Check sheet for the modelled part. Datum: model origin and axes. Units: mm. Face numbers are marked on the shaded views. A direction names the side the tool comes from. Round coordinates to 2 decimals unless told otherwise and drop trailing zeros. Write each loop counter-clockwise with the first axis right and the second up, starting at its lowest first coordinate (ties: lowest second). Pieces come first, ordered by that corner, then holes. Notation, with made-up numbers: M -8,46 L 10,46 A20 cw 10,65 Z; hole C 28,-39.75 d10. An arc over 180 degrees is marked long. Answer in a Markdown table with one row per item.
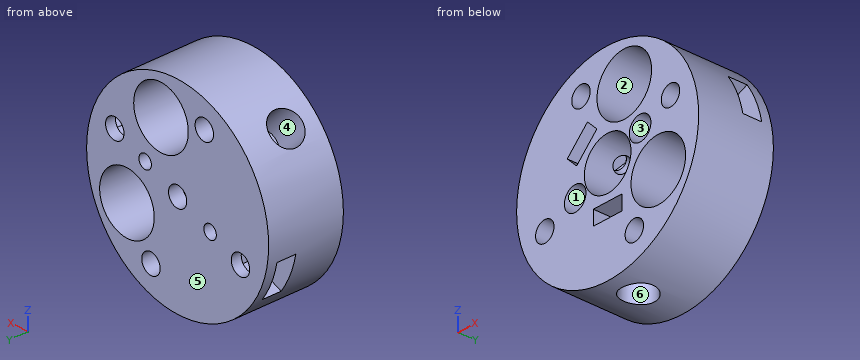
```python
from build123d import *

# Parameters (mm, degrees)
SKETCH1_R               = 20
BOSS_EXTRUDE1_DEPTH     = 7.5
SKETCH4_R               = 5.125
CUT_EXTRUDE2_DEPTH      = 12.15
SKETCH5_R               = 2
CUT_EXTRUDE3_DEPTH      = 1
CUT_EXTRUDE3_DEPTH_BACK = 16
SKETCH2_R               = 2.025
CUT_EXTRUDE1_DEPTH      = 16
CIRPATTERN1_COUNT       = 4
SKETCH6_R               = 1.525
CUT_EXTRUDE4_DEPTH      = 21
CUT_EXTRUDE5_START      = -20
SKETCH7_R               = 3.25
CUT_EXTRUDE5_DEPTH      = 8
CUT_EXTRUDE11_START     = -6.5
CUT_EXTRUDE11_DEPTH     = 2.9
CIRPATTERN2_COUNT       = 2
CIRPATTERN2_ANGLE       = 135
CUT_EXTRUDE7_START      = 5.5
CUT_EXTRUDE7_DEPTH      = 3.8
CIRPATTERN3_COUNT       = 2
CUT_EXTRUDE12_START     = -16.0000001
SKETCH10_R              = 6
CUT_EXTRUDE12_DEPTH     = 17.0000002
CIRPATTERN4_COUNT       = 2
CIRPATTERN4_ANGLE       = 100
CUT_EXTRUDE13_START     = -16.0000001
SKETCH11_R              = 1.375
CUT_EXTRUDE13_DEPTH     = 17.0000002
SKETCH13_R              = 2.375
CUT_EXTRUDE24_DEPTH     = 12
CIRPATTERN5_COUNT       = 2


with BuildPart() as part:
    # Sketch1 → Boss-Extrude1 (new body, symmetric)
    with BuildSketch(Plane(origin=(0, 0, 0), x_dir=(1, 0, 0), z_dir=(0, 1, 0))):
        Circle(SKETCH1_R)
    extrude(amount=BOSS_EXTRUDE1_DEPTH, both=True)

    # Sketch4 → Cut-Extrude2 (cut)
    with BuildSketch(Plane.XZ.offset(7.5)):
        Circle(SKETCH4_R)
    extrude(amount=-CUT_EXTRUDE2_DEPTH, mode=Mode.SUBTRACT)

    # Sketch5 → Cut-Extrude3 (cut, two sides)
    with BuildSketch(Plane(origin=(0, 7.5, 0), x_dir=(1, 0, 0), z_dir=(0, 1, 0))) as cut_extrude3_sk:
        Circle(SKETCH5_R)
    extrude(amount=CUT_EXTRUDE3_DEPTH, mode=Mode.SUBTRACT)
    extrude(cut_extrude3_sk.sketch, amount=-CUT_EXTRUDE3_DEPTH_BACK, mode=Mode.SUBTRACT)

    # Sketch2 → Cut-Extrude1 (cut, through all)
    with BuildSketch(Plane(origin=(0, 7.5, 0), x_dir=(1, 0, 0), z_dir=(0, 1, 0))):
        with Locations((-13.807572802, 5.860966927)):
            Circle(SKETCH2_R)
    cut_extrude1 = extrude(amount=-CUT_EXTRUDE1_DEPTH, mode=Mode.SUBTRACT)

    # CirPattern1: Cut-Extrude1 ×4 about axis
    cirpattern1_axis = Axis((0, 0, 0), (0, 1, 0))
    for i in range(1, CIRPATTERN1_COUNT):
        add(cut_extrude1.rotate(cirpattern1_axis, i * 360 / CIRPATTERN1_COUNT), mode=Mode.SUBTRACT)

    # Sketch6 → Cut-Extrude4 (cut, through all)
    with BuildSketch(Plane.XY):
        with Locations((0, -1.35)):
            Circle(SKETCH6_R)
    cut_extrude4 = extrude(amount=-CUT_EXTRUDE4_DEPTH, mode=Mode.SUBTRACT)

    # Sketch7 → Cut-Extrude5 (cut)
    with BuildSketch(Plane.XY.offset(CUT_EXTRUDE5_START)):
        with Locations((0, -1.35)):
            Circle(SKETCH7_R)
    cut_extrude5 = extrude(amount=CUT_EXTRUDE5_DEPTH, mode=Mode.SUBTRACT)

    # Sketch9 → Cut-Extrude11 (cut)
    with BuildSketch(Plane.XY.offset(CUT_EXTRUDE11_START)):
        Polygon((3.15, -3.168653348), (3.15, 0.468653348), (0, 2.287306696), (-3.15, 0.468653348), (-3.15, -3.168653348), (-3.15, -7.685074736), (3.15, -7.685074736), align=None)
    cut_extrude11 = extrude(amount=-CUT_EXTRUDE11_DEPTH, mode=Mode.SUBTRACT)

    # CirPattern2: Cut-Extrude4, Cut-Extrude5, Cut-Extrude11 ×2 about axis
    cirpattern2_axis = Axis((0, 0, 0), (0, 1, 0))
    for i in range(1, CIRPATTERN2_COUNT):
        add(cut_extrude4.rotate(cirpattern2_axis, i * CIRPATTERN2_ANGLE / (CIRPATTERN2_COUNT - 1)), mode=Mode.SUBTRACT)
        add(cut_extrude5.rotate(cirpattern2_axis, i * CIRPATTERN2_ANGLE / (CIRPATTERN2_COUNT - 1)), mode=Mode.SUBTRACT)
        add(cut_extrude11.rotate(cirpattern2_axis, i * CIRPATTERN2_ANGLE / (CIRPATTERN2_COUNT - 1)), mode=Mode.SUBTRACT)

    # Sketch8 → Cut-Extrude7 (cut)
    with BuildSketch(Plane(origin=(0, 0, 0), x_dir=(1, 0, 0), z_dir=(0, 1, 0)).offset(CUT_EXTRUDE7_START)):
        Polygon((-9.396506885, 3.988580533), (-9.98050566, 8.744868872), (-14.391571577, 10.617255266), (-19.569899143, 12.815324908), (-22.81296751, 5.175134625), (-17.634639943, 2.977064983), (-13.223574027, 1.104678588), align=None)
    cut_extrude7 = extrude(amount=-CUT_EXTRUDE7_DEPTH, mode=Mode.SUBTRACT)

    # CirPattern3: Cut-Extrude7 ×2 about axis
    cirpattern3_axis = Axis((0, 0, 0), (0, 1, 0))
    for i in range(1, CIRPATTERN3_COUNT):
        add(cut_extrude7.rotate(cirpattern3_axis, i * 360 / CIRPATTERN3_COUNT), mode=Mode.SUBTRACT)

    # Sketch10 → Cut-Extrude12 (cut)
    with BuildSketch(Plane(origin=(0, 7.5, 0), x_dir=(1, 0, 0), z_dir=(0, 1, 0)).offset(CUT_EXTRUDE12_START)):
        with Locations((3.654646309, -11.95380945)):
            Circle(SKETCH10_R)
    cut_extrude12 = extrude(amount=CUT_EXTRUDE12_DEPTH, mode=Mode.SUBTRACT)

    # CirPattern4: Cut-Extrude12 ×2 about axis
    cirpattern4_axis = Axis((0, 7.5, 0), (0, 1, 0))
    for i in range(1, CIRPATTERN4_COUNT):
        add(cut_extrude12.rotate(cirpattern4_axis, i * CIRPATTERN4_ANGLE / (CIRPATTERN4_COUNT - 1)), mode=Mode.SUBTRACT)

    # Sketch11 → Cut-Extrude13 (cut)
    with BuildSketch(Plane(origin=(0, 7.5, 0), x_dir=(1, 0, 0), z_dir=(0, 1, 0)).offset(CUT_EXTRUDE13_START)):
        with Locations((7.133912614, -3.028166246)):
            Circle(SKETCH11_R)
    cut_extrude13 = extrude(amount=CUT_EXTRUDE13_DEPTH, mode=Mode.SUBTRACT)

    # Sketch13 → Cut-Extrude24 (cut)
    with BuildSketch(Plane(origin=(0, -7.5, 0), x_dir=(-1, 0, 0), z_dir=(0, -1, 0))):
        with Locations((-7.133912614, -3.028166246)):
            Circle(SKETCH13_R)
    cut_extrude24 = extrude(amount=-CUT_EXTRUDE24_DEPTH, mode=Mode.SUBTRACT)

    # CirPattern5: Cut-Extrude13, Cut-Extrude24 ×2 about axis
    cirpattern5_axis = Axis((0, 0, 0), (0, 1, 0))
    for i in range(1, CIRPATTERN5_COUNT):
        add(cut_extrude13.rotate(cirpattern5_axis, i * 360 / CIRPATTERN5_COUNT), mode=Mode.SUBTRACT)
        add(cut_extrude24.rotate(cirpattern5_axis, i * 360 / CIRPATTERN5_COUNT), mode=Mode.SUBTRACT)


solid = part.part
```
1. Section check B-B, the plane y = -5.25. Count the separate pieces of the cut face and the enclosed holes in it, and give its area (3 significant figures).
Found:
| item | result |
|---|---|
| separate pieces | 1 |
| enclosed holes | 11 |
| area | 824 mm2 |
2. Section check C-C, the plane x = 12.5. Record the cut outline in (y, z).
Found:
| item | result |
|---|---|
| outline | M -7.5,-15.61 L 7.5,-15.61 L 7.5,-11.52 L -7.5,-11.52 Z; M -7.5,0.17 L 7.5,0.17 L 7.5,4.31 L 5.5,4.31 L 5.5,1.65 L 1.7,1.65 L 1.7,4.31 L -7.5,4.31 Z; M -7.5,7.41 L 1.7,7.41 L 1.7,9.81 L 5.5,9.81 L 5.5,7.41 L 7.5,7.41 L 7.5,15.61 L -7.5,15.61 Z |
3. Go/stop test with flat-tipped pins: pin 1 (1.5 mm diameter, centred on x = 8, y = 5.5, fed in from +Z); pin 2 (6 mm diameter, centred on y = 1, z = 6.5, fed in from +X); pin 3 (5 mm diameter, centred on x = -3.5, y = -2, fed in from +Z) (3 decimals). Record where each tip stops, or that it passes through.
Found:
| item | result |
|---|---|
| pin 1 | stops at z = 18.64 |
| pin 2 | stops at x = 19.69 |
| pin 3 | stops at z = 19.975 |
4. Scan lines: L1, parallel to Y at x = 16, z = 7; L2, parallel to Z at x = 2, y = 0.25; L3, parallel to Z at x = 16, y = 4.5. Record each from-to range of solid material in increasing order.
Found:
| item | result |
|---|---|
| L1 | y = -7.5 to 1.7, 5.5 to 7.5 |
| L2 | z = -12 to -9.4, -6.5 to -4.72, 4.72 to 6.19, 17.72 to 19.9 |
| L3 | z = -12 to -9.19, -2.16 to 2.28, 11.3 to 12 |
5. Access from +Z, -Z, +X, -X, +Y, -Y to the whole of each face (thin tool, end or side, straight path). Record for the marked faces 1 and 2.
Found:
| item | result |
|---|---|
| face 1 | -Y |
| face 2 | +Y, -Y |
6. Section check A-A, the plane z = -15. Record the cut outline in (x, y).
Found:
| item | result |
|---|---|
| outline | M -13.23,-7.5 L 4.22,-7.5 L 4.22,7.5 L -13.23,7.5 Z; M 7.5,-7.5 L 13.23,-7.5 L 13.23,7.5 L 7.5,7.5 Z; hole C 0,-1.35 d6.5 |
7. Draft check along Y on the marked faces 3, 4, 5 and 6. Enter one of: +Y half, -Y half, draft (parallel to the pull), parting line (faces both ways), or undercut.
Found:
| item | result |
|---|---|
| face 3 | draft |
| face 4 | undercut |
| face 5 | +Y half |
| face 6 | undercut |
